from build123d import *

# Parameters (mm, degrees)
SLOT_CUT_EXTRUDE1_DEPTH      = 13.826535018
SLOT_CUT_EXTRUDE1_DEPTH_BACK = 13.826535018
SKETCH2_W                    = 0.6
SKETCH2_H                    = 0.8
SKETCH11_W                   = 2.1
SKETCH11_H                   = 0.25
POINT_CUT_EXTRUDE8_DEPTH     = 13.82653504


with BuildPart() as part:
    # Sketch1 → base-Revolve (revolve)
    with BuildSketch(Plane.XY, mode=Mode.PRIVATE) as base_revolve_sk:
        with BuildLine():
            Line((0, 0), (0, 1.6))
            ThreePointArc((0, 1.6), (0.351471863, 2.448528137), (1.2, 2.8))
            Line((1.2, 2.8), (2.2, 2.8))
            Line((2.2, 2.8), (2.2, 1.3))
            ThreePointArc((2.2, 1.3), (2.229289322, 1.229289322), (2.3, 1.2))
            Line((2.3, 1.2), (2.9, 1.2))
            Line((2.9, 1.2), (3.2, 1.5))
            Line((3.2, 1.5), (12.2, 1.5))
            Line((12.2, 1.5), (12.2, 0))
            Line((12.2, 0), (0, 0))
        make_face()
    revolve(base_revolve_sk.sketch.rotate(Axis((0, 0, 0), (1, 0, 0)), 90), axis=Axis((0, 0, 0), (1, 0, 0)))

    # Sketch2 → slot_Cut-Extrude1 (cut, two sides: drawn at the far end of the back side and taken through both)
    with BuildSketch(Plane.XY.offset(-SLOT_CUT_EXTRUDE1_DEPTH_BACK)):
        with Locations((0.3, 0)):
            Rectangle(SKETCH2_W, SKETCH2_H)
    extrude(amount=SLOT_CUT_EXTRUDE1_DEPTH + SLOT_CUT_EXTRUDE1_DEPTH_BACK, mode=Mode.SUBTRACT)

    # Sketch8 → point_Cut-Revolve1 (revolve, cut)
    with BuildSketch(Plane.XY, mode=Mode.PRIVATE) as point_cut_revolve1_sk:
        Polygon((12.2, 0), (12.708, 0), (12.708, 2.008), (11.611102725, 2.008), (11.611102725, 1.5), (12.2, 1.16), align=None)
    revolve(point_cut_revolve1_sk.sketch.rotate(Axis((0, 0, 0), (1, 0, 0)), 90), axis=Axis((0, 0, 0), (1, 0, 0)), mode=Mode.SUBTRACT)

    # Sketch11 → point_Cut-Extrude8 (cut, through all)
    with BuildSketch(Plane.XY):
        with Locations((11.15, -0.125)):
            Rectangle(SKETCH11_W, SKETCH11_H)
    extrude(amount=POINT_CUT_EXTRUDE8_DEPTH, mode=Mode.SUBTRACT)


solid = part.part
Work out the finished part from the listing and answer in its coordinate system (mm). A direction names the side the tool comes from. Coordinates: 2 decimals unless noted, no trailing zeros. Write each loop counter-clockwise with the first axis right and the second up, starting at its lowest first coordinate (ties: lowest second). Pieces come first, ordered by that corner, then holes.
1. Consider line 1 along X through (y, z) = (0.3, 2.3); line 2 along X through (y, z) = (0.05, -0.1); line 3 along X through (y, z) = (0, -1.3). Determine where each line is inside the solid, lowest interval first.
Results list:
line 1: x = 0.6 to 2.2
line 2: x = 0.6 to 12.2
line 3: x = 0.6 to 2.2, 3 to 11.96
2. Flat-ended cylindrical pins translate along their axes: pin 1 (1 mm diameter, centred on x = 3, z = 0, fed in from +Y); pin 2 (1.5 mm diameter, centred on x = 4, z = -2, fed in from -Y); pin 3 (0.6 mm diameter, centred on y = 0, z = 0.5, fed in from -X). Find the tip coordinate at first contact, or state that the pin passes through.
Results list:
pin 1: stops at y = 1.5
pin 2: stops at y = -0.83
pin 3: stops at x = 0.6
3. For a pull along X with two mould halves and no side action, classify faces 4 (the flat face through (11, -0.25, 1)), 5 (the flat face through (0.6, 0, 0)), 6 (the cylindrical face through (2.6, -1.01, 0.65)), 7 (the flat face through (12.2, 0.2, 0)) as +X half, -X half, draft (parallel to the pull), parting line (faces both ways), or undercut.
Results list:
face 4: draft
face 5: -X half
face 6: undercut
face 7: +X half
4. The part is cut by section B-B, the plane x = 8.25. Write down the section's boundary in (y, z).
Results list:
outline: circle Ø3 at (0, 0)
5. For faces 1 (the flat face through (0, -1, 0)), 2 (the flat face through (11, 0, 1)), 3 (the cylindrical face through (7.46, -0.45, 1.43)), determine the directions among +Z, -Z, +X, -X, +Y, -Y from which every point of the face is accessible in a straight line to the end or side of a thin tool.
Results list:
face 1: +Z, -Z, -X, +Y, -Y
face 2: +Z, +X
face 3: +X
6. The part is cut by section A-A, the plane x = 2. Write down the section's boundary in (y, z).
Results list:
outline: circle Ø5.6 at (0, 0)
